```python
from build123d import *

# Parameters (mm, degrees)
F0_R     = 5
F1_DEPTH = 15


with BuildPart() as f1:
    # F0 (on Front) → F1 (new body)
    with BuildSketch(Plane.XZ):
        with BuildLine():
            ThreePointArc((0, 75), (-24.748737, 64.748737), (-35, 40))
            Line((-35, 40), (-35, 0))
            Line((-35, 0), (-35, -40))
            ThreePointArc((-35, -40), (-24.748737, -64.748737), (0, -75))
            ThreePointArc((0, -75), (24.748737, -64.748737), (35, -40))
            Line((35, -40), (35, 0))
            Line((35, 0), (35, 40))
            ThreePointArc((35, 40), (24.748737, 64.748737), (0, 75))
        make_face()
        with Locations((-17.67767, -57.67767)):
            Circle(F0_R, mode=Mode.SUBTRACT)
        with Locations((-25, -40)):
            Circle(F0_R, mode=Mode.SUBTRACT)
        with Locations((-25, -20)):
            Circle(F0_R, mode=Mode.SUBTRACT)
        with Locations((0, -65)):
            Circle(F0_R, mode=Mode.SUBTRACT)
        with Locations((17.67767, -57.67767)):
            Circle(F0_R, mode=Mode.SUBTRACT)
        with Locations((25, -40)):
            Circle(F0_R, mode=Mode.SUBTRACT)
        with Locations((25, -20)):
            Circle(F0_R, mode=Mode.SUBTRACT)
        with Locations((-25, 0)):
            Circle(F0_R, mode=Mode.SUBTRACT)
        with Locations((-25, 20)):
            Circle(F0_R, mode=Mode.SUBTRACT)
        with Locations((-25, 40)):
            Circle(F0_R, mode=Mode.SUBTRACT)
        with Locations((-17.67767, 57.67767)):
            Circle(F0_R, mode=Mode.SUBTRACT)
        with BuildLine():
            ThreePointArc((-15, 40), (-10.606602, 50.606602), (0, 55))
            ThreePointArc((0, 55), (10.606602, 50.606602), (15, 40))
            Line((15, 40), (15, 0))
            Line((15, 0), (15, -40))
            ThreePointArc((15, -40), (10.606602, -50.606602), (0, -55))
            ThreePointArc((0, -55), (-10.606602, -50.606602), (-15, -40))
            Line((-15, -40), (-15, 0))
            Line((-15, 0), (-15, 40))
        make_face(mode=Mode.SUBTRACT)
        with Locations((25, 0)):
            Circle(F0_R, mode=Mode.SUBTRACT)
        with Locations((25, 20)):
            Circle(F0_R, mode=Mode.SUBTRACT)
        with Locations((0, 65)):
            Circle(F0_R, mode=Mode.SUBTRACT)
        with Locations((25, 40)):
            Circle(F0_R, mode=Mode.SUBTRACT)
        with Locations((17.67767, 57.67767)):
            Circle(F0_R, mode=Mode.SUBTRACT)
    extrude(amount=F1_DEPTH)


solid = f1.part
```
The listing builds one solid part. Answer for the finished solid, in the listing's coordinates (mm). A direction names the side the tool comes from. Give positions to 0.01 mm unless a question says otherwise; leave off trailing zeros. Order: outer loops, then holes, each group sorted by start corner. A loop starts at its lowest first (then second) coordinate and runs counter-clockwise, first axis right, second up.
Item 1: The part is cut by section D-D, the plane z = 65. Give the vertices of the cut face in (x, y).
From the geometry:
outline: (-24.49, -15) - (-5, -15) - (-5, 0) - (-24.49, 0) - close; (5, -15) - (24.49, -15) - (24.49, 0) - (5, 0) - close
Item 2: Which of the six approach directions +Z, -Z, +X, -X, +Y, -Y give full straight-line access (tool end or side, diameter ignored) to faces 1 (the face through (-15, -7, -1)), 2 (the face through (-35, -7, 1))?
From the geometry:
face 1: +Y, -Y
face 2: +Z, -Z, -X, +Y, -Y
Item 3: The part is cut by section B-B, the plane x = -25. Give the vertices of the cut face in (y, z).
From the geometry:
outline: (-15, -64.49) - (0, -64.49) - (0, -45) - (-15, -45) - close; (-15, -35) - (0, -35) - (0, -25) - (-15, -25) - close; (-15, -15) - (0, -15) - (0, -5) - (-15, -5) - close; (-15, 5) - (0, 5) - (0, 15) - (-15, 15) - close; (-15, 25) - (0, 25) - (0, 35) - (-15, 35) - close; (-15, 45) - (0, 45) - (0, 64.49) - (-15, 64.49) - close
Item 4: The part is cut by section C-C, the plane x = -3.5. Give the vertices of the cut face in (y, z).
From the geometry:
outline: (-15, -74.82) - (0, -74.82) - (0, -68.57) - (-15, -68.57) - close; (-15, -61.43) - (0, -61.43) - (0, -54.59) - (-15, -54.59) - close; (-15, 54.59) - (0, 54.59) - (0, 61.43) - (-15, 61.43) - close; (-15, 68.57) - (0, 68.57) - (0, 74.82) - (-15, 74.82) - close
Item 5: Find the intervals of material crossed by probe 1 along X at (y, z) = (-3.5, 8.5); probe 2 along X at (y, z) = (-14, 39.5); probe 3 along Z at (x, y) = (-25.5, -10.25), in increasing order.
From the geometry:
probe 1: x = -35 to -15, 15 to 35
probe 2: x = -35 to -29.97, -20.03 to -15, 15 to 20.03, 29.97 to 35
probe 3: z = -63.97 to -44.97, -35.03 to -24.97, -15.03 to -4.97, 4.97 to 15.03, 24.97 to 35.03, 44.97 to 63.97
Item 6: For a pull along X with two mould halves and no side action, classify faces 3 (the face through (-16, 0, 1)), 4 (the face through (-22.673, -7.395, -57.458)), 5 (the face through (35, -7, -1)) as pulls with the +X half, pulls with the -X half, needs draft (parallel to the pull), parting line crosses it, or undercut.
From the geometry:
face 3: needs draft
face 4: undercut
face 5: pulls with the +X half
Item 7: Given pin 1 Ø9 at (x, z) = (25, 40) entering from +Y; pin 2 Ø1 at (x, y) = (15, -6) entering from +Z; pin 3 Ø1 at (x, y) = (-4.5, -2) entering from -Z; pin 4 Ø2 at (y, z) = (-9.5, -57) entering from -X, each flat-ended and moving along its own axis, determine where each tip first touches the part or whether it passes through.
From the geometry:
pin 1: passes through
pin 2: stops at z = 71.86
pin 3: stops at z = -74.77
pin 4: stops at x = -31.13
Item 8: The part is cut by section A-A, the plane z = 0. Give the vertices of the cut face in (x, y), and give its area (3 significant figures).
From the geometry:
outline: (-35, -15) - (-30, -15) - (-30, 0) - (-35, 0) - close; (-20, -15) - (-15, -15) - (-15, 0) - (-20, 0) - close; (15, -15) - (20, -15) - (20, 0) - (15, 0) - close; (30, -15) - (35, -15) - (35, 0) - (30, 0) - close
area: 300 mm2
